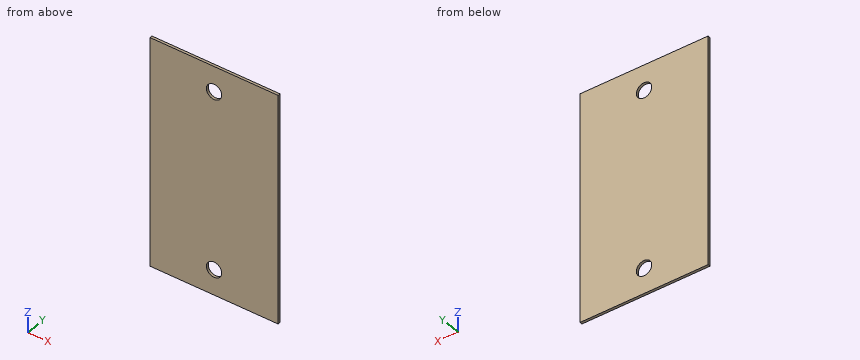
Autodesk Inventor part; units mm, degrees
ref_plane "YZ Plane" through (0, 0, 0) normal (1, 0, 0) x (0, 1, 0)
ref_plane "XZ Plane" through (0, 0, 0) normal (0, 1, 0) x (-1, 0, 0)
ref_plane "XY Plane" through (0, 0, 0) normal (0, 0, 1) x (1, 0, 0)
sketch "Sketch1" plane through (0, 0, 0) normal (0, 1, 0) x (-1, 0, 0)
  line L0 (125, 225) -> (-125, 225)
  line L1 (-125, 225) -> (-125, -225)
  line L2 (-125, -225) -> (125, -225)
  line L3 (125, -225) -> (125, 225)
  line L4 (125, 225) -> (-125, -225) construction
  line L5 (-125, 225) -> (125, -225) construction
  point P0 (0, 0)
  dimension "d0" = 250
  dimension "d1" = 450
extrude "Extrusion1" add sketch "Sketch1" along normal blind 5
sketch "Sketch2" plane through (0, 0, 0) normal (0, -1, 0) x (1, 0, 0)
  circle A0 centre (0, 175) radius 15
  line L0 (-125, 225) -> (125, 225)
  line L1 (-125, 0) -> (125, 0) construction
  line L2 (125, 225) -> (125, -225) construction
  circle A1 centre (0, -175) radius 15
  point P0 (0, 0)
  dimension "d4" = 30
  dimension "d5" = 50
extrude "Extrusion2" cut sketch "Sketch2" against normal blind 5
equation "\"d0\" = boxl"
equation "\"d1\" = boxw"
equation "\"d2\" = pvct"
equation "\"d6\" = pvct"
equation "\"solhole\" = 3"
equation "\"solholespacing\" = 16"
equation "\"ssolw\" = 63"
equation "\"bsoll\" = 126"
equation "\"bsolw\" = 91"
equation "\"bsolh\" = 126"
equation "\"tapl\" = 31"
equation "\"tl\" = 32"
equation "\"eloboww\" = 25"
equation "\"pvct\" = 5"
equation "\"boxw\" = 450"
equation "\"boxl\" = 250"
equation "\"boxh\" = 258"
equation "\"supporth\" = 15"
equation "\"play\" = 0.5"
equation "\"arw\" = 54"
equation "\"arl\" = 102"
equation "\"psuh\" = 85"
equation "\"screenw\" = 197"
equation "\"screenl\" = 115"
equation "\"pcbw\" = 76"
equation "\"pcbl\" = 86"
equation "\"pcbh\" = 46"
equation "\"seph\" = 105"
equation "\"diapowerouter\" = 25"
equation "\"dialoadouter\" = 25"
equation "\"diaetape\" = 25"
equation "\"distpumps\" = 75"
equation "\"diaph\" = 32"
equation "\"diaetapeouter\" = 36"
equation "\"diaphouter\" = 48"
equation "\"diaload\" = 16"
equation "\"distbubblewater\" = 82"
equation "\"diapower\" = 16"
equation "\"pumpinner\" = 16"
equation "\"airoutouter\" = 39"
equation "\"airinouter\" = 39"
equation "\"waterouter\" = 39"
equation "\"airininner\" = 28"
equation "\"waterinner\" = 28"
equation "\"airoutinner\" = 28"
equation "\"pumpouter\" = 25"
properties part number "sb_bottom" material "PVC-Piping"
Geometry check sheet. Reference: the model listing, model coordinates, mm. Round coordinates to 2 decimals unless told otherwise and drop trailing zeros. Loops run counter-clockwise (first coordinate to the right, second up) from the corner with the lowest first, then second, coordinate; pieces in that order, holes last. Notation, with made-up numbers: (12, 60.25) -> (53, 60.25) arc R25 ccw to (53, 76.25) -> close; hole circle Ø2 at (71, 7.5). An arc over 180 degrees is marked (long way). Use a Markdown table: item, result.
(1) Go/stop test with a flat-tipped pin: P1, Ø8, axis at x = -80.5, z = 92, coming from the -Y side. Record where the tip stops, or that it passes through.
Calculated:
| item | result |
|---|---|
| P1 | y = 0 |
(2) Sectioned sample at A-A (z = -175). Enter the section's corners in (x, y).
Calculated:
| item | result |
|---|---|
| outline | (-125, 0) -> (-15, 0) -> (-15, 5) -> (-125, 5) -> close; (15, 0) -> (125, 0) -> (125, 5) -> (15, 5) -> close |
(3) Scan lines: probe 1 along Z at (x, y) = (0, 2.3); probe 2 along Z at (x, y) = (2.5, 4.65); probe 3 along X at (y, z) = (2.8, 163). Record each from-to range of solid material in increasing order.
Calculated:
| item | result |
|---|---|
| probe 1 | -225 to -190, -160 to 160, 190 to 225 |
| probe 2 | -225 to -189.79, -160.21 to 160.21, 189.79 to 225 |
| probe 3 | -125 to -9, 9 to 125 |
(4) Sectioned sample at B-B (x = 0). Enter the section's corners in (y, z).
Calculated:
| item | result |
|---|---|
| outline | (0, -225) -> (5, -225) -> (5, -190) -> (0, -190) -> close; (0, -160) -> (5, -160) -> (5, 160) -> (0, 160) -> close; (0, 190) -> (5, 190) -> (5, 225) -> (0, 225) -> close |
